Print and shaded views of the part. All mm, measured from the part's lowest x, y and z. A direction names the side the tool comes from. Coordinates: 2 decimals unless noted, no trailing zeros. Order: outer loops, then holes, each group sorted by start corner. A loop starts at its lowest first (then second) coordinate and runs counter-clockwise, first axis right, second up. Notation, with made-up numbers: (57, 17) -> (112, 17) arc R22 ccw to (112, 36) -> close; hole circle Ø2 at (-26, -34). An arc over 180 degrees is marked (long way). Use one line per item in the form item = value. Start each with the question number.
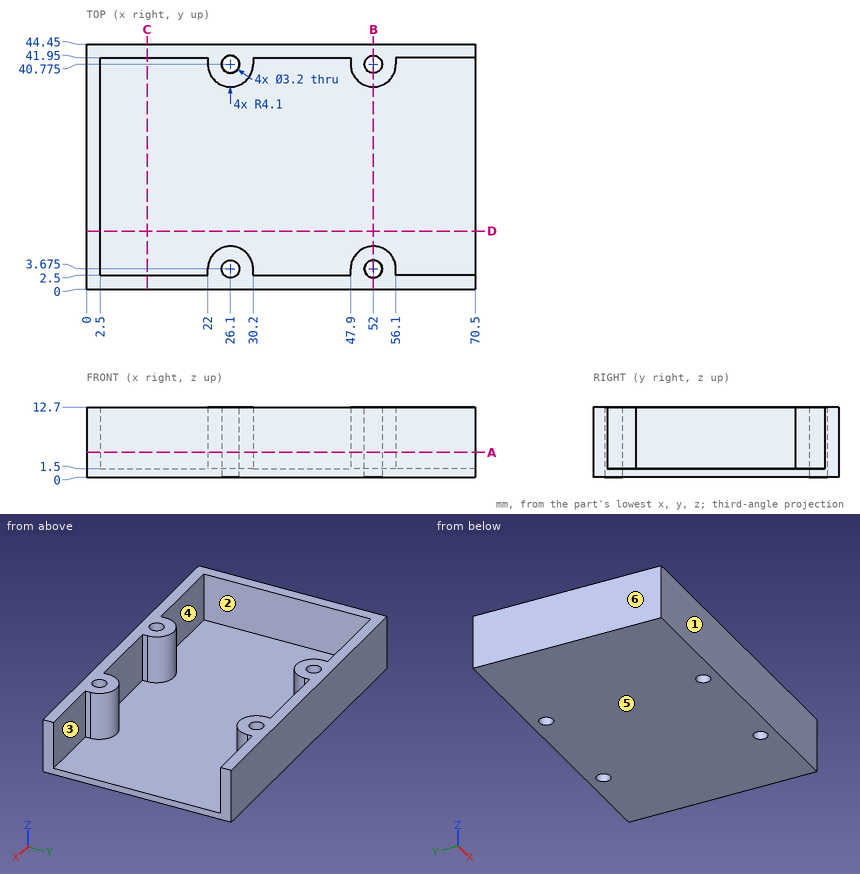
1) 3-axis set-ups, long thin cutter, end or side, ignore diameter. For the marked faces 1, 2 and 3: which of +Z, -Z, +X, -X, +Y, -Y reach the whole face in a straight line?
2) Drop flat-ended pins along their axis: P1, Ø6, axis at y = 37, z = 9.5, coming from the +X side; P2, Ø0.6, axis at y = 3, z = 8, coming from the +X side; P3, Ø2, axis at x = 48, y = 36.5, coming from the +Z side; P4, Ø3, axis at x = 52, y = 3.675, coming from the +Z side. Give the stop position or say it passes through.
3) Cut at D-D on y = 10.5. Give the cut face in (x, z).
4) Cut at C-C on x = 11. Give the cut face in (y, z), then the cut area to 3 significant figures.
5) Cut at B-B on x = 52. Give the cut face in (y, z) (3 decimals).
6) Cut at A-A on z = 4.5. Give the cut face in (x, y) (3 decimals), then the cut area to 3 significant figures.
7) Two-plate mould, pull along X, no slides. Class the marked faces 4, 5 and 6: released by +X, released by -X, zero draft, split by the parting line, or undercut.
8) Probe L1, parallel to Y at x = 52, z = 7.25 (3 decimals); L2, parallel to X at y = 37, z = 2.75; L3, parallel to Y at x = 33, z = 5. List the from-to ranges inside material, lowest first.
Values follow:
q1.face_1 = +Z, -Z, +X, -X, -Y
q1.face_2 = +Z
q1.face_3 = +Z, +X
q2.P1 = 56.03
q2.P2 = 56.1
q2.P3 = 1.5
q2.P4 = through
q3.outline = (0, 0) -> (70.5, 0) -> (70.5, 1.5) -> (2.5, 1.5) -> (2.5, 12.7) -> (0, 12.7) -> close
q4.outline = (0, 0) -> (44.45, 0) -> (44.45, 12.7) -> (41.95, 12.7) -> (41.95, 1.5) -> (2.5, 1.5) -> (2.5, 12.7) -> (0, 12.7) -> close
q4.area = 123 mm^2
q5.outline = (0, 0) -> (2.075, 0) -> (2.075, 12.7) -> (0, 12.7) -> close; (5.275, 0) -> (39.175, 0) -> (39.175, 12.7) -> (36.675, 12.7) -> (36.675, 1.5) -> (7.775, 1.5) -> (7.775, 12.7) -> (5.275, 12.7) -> close; (42.375, 0) -> (44.45, 0) -> (44.45, 12.7) -> (42.375, 12.7) -> close
q6.outline = (0, 0) -> (70.5, 0) -> (70.5, 2.5) -> (56.1, 2.5) -> (56.1, 3.675) arc R4.1 ccw to (47.9, 3.675) -> (47.9, 2.5) -> (30.2, 2.5) -> (30.2, 3.675) arc R4.1 ccw to (22, 3.675) -> (22, 2.5) -> (2.5, 2.5) -> (2.5, 41.95) -> (22, 41.95) -> (22, 40.775) arc R4.1 ccw to (30.2, 40.775) -> (30.2, 41.95) -> (47.9, 41.95) -> (47.9, 40.775) arc R4.1 ccw to (56.1, 40.775) -> (56.1, 41.95) -> (70.5, 41.95) -> (70.5, 44.45) -> (0, 44.45) -> close; hole circle Ø3.2 at (26.1, 3.675); hole circle Ø3.2 at (26.1, 40.775); hole circle Ø3.2 at (52, 3.675); hole circle Ø3.2 at (52, 40.775)
q6.area = 563 mm^2
q7.face_4 = undercut
q7.face_5 = zero draft
q7.face_6 = released by -X
q8.L1 = 0 to 2.075, 5.275 to 7.775, 36.675 to 39.175, 42.375 to 44.45
q8.L2 = 0 to 2.5, 24.5 to 27.7, 50.4 to 53.6
q8.L3 = 0 to 2.5, 41.95 to 44.45
